Autodesk Inventor part; units mm, degrees
ref_plane "YZ Plane" through (0, 0, 0) normal (1, 0, 0) x (0, 1, 0)
ref_plane "XZ Plane" through (0, 0, 0) normal (0, 1, 0) x (-1, 0, 0)
ref_plane "XY Plane" through (0, 0, 0) normal (0, 0, 1) x (1, 0, 0)
sketch "Sketch1" plane through (0, 0, 0) normal (0, 1, 0) x (-1, 0, 0)
  circle A0 centre (0, 0) radius 5.4
  dimension "d0" = 10.8
extrude "Extrusion1" add sketch "Sketch1" along normal blind 3
fillet "Fillet1" radius 1 1 edges at (5.4, 3, 0)
sketch "Sketch2" plane through (0, 3, 0) normal (0, 1, 0) x (1, 0, 0)
  circle A0 centre (0, 0) radius 4.25
  dimension "d4" = 8.5
extrude "Extrusion2" add sketch "Sketch2" along normal blind 6.8
sketch "Sketch3" plane through (0, 0, 0) normal (0, -1, 0) x (1, 0, 0)
  circle A0 centre (0, 0) radius 3.5
  dimension "d7" = 7
extrude "Extrusion3" add sketch "Sketch3" along normal blind 5.9
sketch "Sketch4" plane through (0, -5.9, 0) normal (0, -1, 0) x (1, 0, 0)
  circle A0 centre (0, 0) radius 4.25
  circle A1 centre (0, 0) radius 3.83
  dimension "d10" = 7.66
extrude "Extrusion4" add sketch "Sketch4" against normal blind 4 contours A1
sketch "Sketch5" plane through (0, 9.8, 0) normal (0, 1, 0) x (1, 0, 0)
  line L0 (-3.9765, 1.5) -> (-3.4765, 1.5)
  line L1 (-3.4765, 1.5) -> (-3.4765, -1.5)
  line L2 (-3.4765, -1.5) -> (-3.9765, -1.5)
  line L3 (-3.9765, -1.5) -> (-3.9765, 1.5)
  circle A0 centre (0, 0) radius 4.25
  line L4 (-1.5, -3.9765) -> (-1.5, -3.4765)
  line L5 (-1.5, -3.4765) -> (1.5, -3.4765)
  line L6 (1.5, -3.4765) -> (1.5, -3.9765)
  line L7 (1.5, -3.9765) -> (-1.5, -3.9765)
  line L8 (3.9765, -1.5) -> (3.4765, -1.5)
  line L9 (3.4765, -1.5) -> (3.4765, 1.5)
  line L10 (3.4765, 1.5) -> (3.9765, 1.5)
  line L11 (3.9765, 1.5) -> (3.9765, -1.5)
  dimension "d13" = 0.5
  dimension "d14" = 3
  dimension "d17" = 180
extrude "Extrusion5" add sketch "Sketch5" along normal blind 6 contours L0 L1 L2 L3 | L11 L8 L9 L10 | L4 L5 L6 L7
fillet "Fillet2" radius 1.5 6 edges at (3.7265, 15.8, -1.5) (3.7265, 15.8, 1.5) (1.5, 15.8, 3.7265) (-1.5, 15.8, 3.7265) (-3.7265, 15.8, 1.5) (-3.7265, 15.8, -1.5)
chamfer "Chamfer1" distance 0.3 angle 45 1 edges at (-3.83, -1.9, 0)
chamfer "Chamfer2" distance 0.3 angle 45 1 edges at (-3.83, -5.9, 0)
sketch "Sketch6" plane through (0, -5.9, 0) normal (0, -1, 0) x (1, 0, 0)
  circle A0 centre (0, 0) radius 3.83
  circle A1 centre (0, 0) radius 2.83
  dimension "d28" = 1
extrude "Extrusion6" cut sketch "Sketch6" against normal blind 8 contours A1
sketch "Sketch7" plane through (0, 2.1, 0) normal (0, -1, 0) x (1, 0, 0)
  circle A0 centre (0, 0) radius 1.1
  dimension "d31" = 2.2
extrude "Extrusion7" add sketch "Sketch7" along normal blind 5.5
fillet "Fillet3" radius 1.1 1 edges at (-1.1, -3.4, 0)
equation "\"d34\" = 0.5 * d31"
properties part number "gniazdo_zasilania"
The model under review builds one solid part; all positions refer to its coordinate system, in mm. A direction names the side the tool comes from. Give positions to 0.01 mm unless a question says otherwise; leave off trailing zeros. Order: outer loops, then holes, each group sorted by start corner. A loop starts at its lowest first (then second) coordinate and runs counter-clockwise, first axis right, second up. Notation, with made-up numbers: (18.25, 70) - (56.25, 70) arc R21 cw to (56.25, 78) - close; hole circle Ø1 at (-5.75, 71). An arc over 180 degrees is marked (long way). Use CSV: the item, a comma, the result in double quotes. Start each with the question number.
Q1. We need section B-B, the plane y = 0.5. Write out the cut boundary in (x, z).
Q2. The part is to be moulded in two halves that separate along Y. For faces 1 (the flat face through (3.976, 13, 0)), 2 (the cylindrical face through (3.233, -0.937, 1.341)), 3 (the flat face through (1, 2.1, -1)), say which applies: +Y half, -Y half, draft (parallel to the pull), parting line (faces both ways), or undercut.
Q3. We need section A-A, the plane y = 14. Write out the cut boundary in (x, z).
Q4. Tool access review of faces 4 (the flat face through (-3.976, 13, 0)), 5 (the flat face through (-3.476, 13, 0)), 6 (the cylindrical face through (2.285, 6.352, 3.584)), 7 (the cylindrical face through (1.05, -0.07, -0.33)): name each direction out of +Z, -Z, +X, -X, +Y, -Y from which nothing blocks a thin tool from reaching the whole face with its end or side.
Q5. Clearance check with flat-ended pins moving along their axes: pin 1 Ø2.5 at (y, z) = (12, -0.5) entering from -X; pin 2 Ø4 at (x, y) = (-3.5, 9) entering from +Z; pin 3 Ø0.9 at (y, z) = (14, 0.5) entering from +X. State where each tip first meets the part, or that it passes through.
Q6. We need section C-C, the plane y = 8.5. Write out the cut boundary in (x, z).
Q7. To check wall thickness, follow line 1 along Z through (x, y) = (0, -1); line 2 along Z through (x, y) = (0, -3); line 3 along X through (y, z) = (5, -1.5). State the ranges of each line that lie inside material, in increasing order. Write a range as [from, to].
Outcome:
1,outline,"circle Ø10.8 at (0, 0); circle Ø2.2 at (0, 0); hole circle Ø5.66 at (0, 0)"
2,face 1,"draft"
2,face 2,"undercut"
2,face 3,"-Y half"
3,outline,"(-3.98, -1.5) - (-3.48, -1.5) - (-3.48, 1.5) - (-3.98, 1.5) - close; (-1.5, 3.48) - (1.5, 3.48) - (1.5, 3.98) - (-1.5, 3.98) - close; (3.48, -1.5) - (3.98, -1.5) - (3.98, 1.5) - (3.48, 1.5) - close"
4,face 4,"+Z, -Z, -X, +Y"
4,face 5,"+Z, -Z, +Y"
4,face 6,"+Y"
4,face 7,"-Y"
5,pin 1,"stops at x = -3.98"
5,pin 2,"stops at z = 3.98"
5,pin 3,"stops at x = 3.98"
6,outline,"circle Ø8.5 at (0, 0)"
7,line 1,"z = [-3.5, -2.83], [-1.1, 1.1], [2.83, 3.5]"
7,line 2,"z = [-3.83, -2.83], [-0.85, 0.85], [2.83, 3.83]"
7,line 3,"x = [-3.98, 3.98]"
